from build123d import *

# Parameters (mm, degrees)
ESQUISSE1_R        = 15
BOSS_EXTRU_1_DEPTH = 15
CONG_1_R           = 10
ESQUISSE3_R        = 10
BOSS_EXTRU_2_DEPTH = 80


with BuildPart() as part:
    # Esquisse1 → Boss.-Extru.1 (new body)
    with BuildSketch(Plane(origin=(0, 0, 0), x_dir=(1, 0, 0), z_dir=(0, 1, 0))):
        Circle(ESQUISSE1_R)
    extrude(amount=BOSS_EXTRU_1_DEPTH)

    # Congé1
    cong_1_edges = [part.edges().sort_by_distance(p)[0] for p in [
        (-15, 15, 0),
    ]]
    fillet(cong_1_edges, radius=CONG_1_R)

    # Esquisse3 → Boss.-Extru.2 (add)
    with BuildSketch(Plane.XZ):
        Circle(ESQUISSE3_R)
    extrude(amount=BOSS_EXTRU_2_DEPTH)


solid = part.part
Here's how the part is built. I have some questions about the finished solid (model axes, mm). A direction names the side the tool comes from. Coordinates: 2 decimals unless noted, no trailing zeros. Loops run counter-clockwise (first coordinate to the right, second up) from the corner with the lowest first, then second, coordinate; pieces in that order, holes last. Notation, with made-up numbers: (38.5, 79.5) -> (65.5, 79.5) arc R18 cw to (65.5, 106.5) -> close; hole circle Ø9 at (-29, 56.25). An arc over 180 degrees is marked (long way). Use one line per item in the form item = value. Start each with the question number.
(1) Will these pins go through, and if not, where does the flat tip stop? pin 1 (6 mm diameter, centred on x = -6.5, y = -11, fed in from -Z); pin 2 (8 mm diameter, centred on x = 5, y = -63.5, fed in from -Z); pin 3 (8 mm diameter, centred on x = 4.5, y = -43.5, fed in from -Z).
(2) On a 3-axis mill with a long thin cutter (end or side, diameter ignored), from which of +Z, -Z, +X, -X, +Y, -Y can I reach the whole of each face in a straight line? I mean faces 3 (the face through (0, -80, 0)), 4 (the face through (-2.17, -39.44, -9.76)). Say none if no direction works.
(3) We'd pull the mould along Z, two halves only. Please class faces 1 (the face through (-14.985, 2.465, -0.66)), 2 (the face through (3, 0, 10)): pulls with the +Z half, pulls with the -Z half, needs draft (parallel to the pull), parting line crosses it, or undercut.
(4) If we section it at A-A (y = 3.5): Please give me the cut outline in (x, z), then the cut area to 3 significant figures.
(5) If we section it at B-B (y = -26.5): Please give me the cut outline in (x, z), then the cut area to 3 significant figures.
(6) Please list where these lines run through material, in increasing order: line 1 along Z through (x, y) = (0, -57); line 2 along X through (y, z) = (-39.5, -5.75); line 3 along X through (y, z) = (-33, 0.5).
Verdict:
q1.pin_1 = -9.37
q1.pin_2 = -9.95
q1.pin_3 = -9.99
q2.face_3 = +Z, -Z, +X, -X, -Y
q2.face_4 = -Y
q3.face_1 = parting line crosses it
q3.face_2 = needs draft
q4.outline = circle Ø30 at (0, 0)
q4.area = 707 mm²
q5.outline = circle Ø20 at (0, 0)
q5.area = 314 mm²
q6.line_1 = -10 to 10
q6.line_2 = -8.18 to 8.18
q6.line_3 = -9.99 to 9.99
